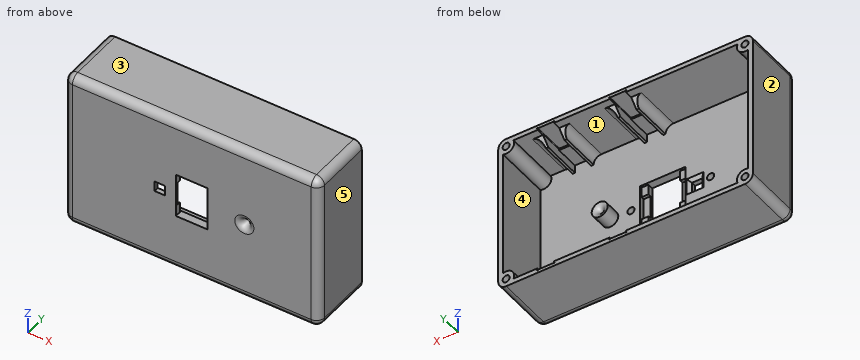
from build123d import *

# Parameters (mm, degrees)
SKETCH1_W                    = 160
SKETCH1_H                    = 100
MAINBODY_DEPTH               = 40
FILLET1_R                    = 5
SHELL1_START                 = 5
SHELL1_DEPTH                 = 35
ROTARYASSEMBLYCUTOUTSKETCH_W = 10.2
ROTARYASSEMBLYCUTOUTSKETCH_H = 20
ROTARYASSEMBLYCUTOUT_DEPTH   = 1
SKETCH5_R                    = 5
SCREWHOLEMATERIAL_DEPTH      = 35
SKETCH6_R                    = 2.25
INSERTHOLE_DEPTH             = 10
SKETCH8_W                    = 20
SKETCH8_H                    = 28
SCREENCUTOUT_DEPTH           = 101.623058987
SKETCH7_W                    = 28.6
SKETCH7_H                    = 28
SCREENCUTOUT1_DEPTH          = 1.4
SKETCH9_W                    = 28.6
SKETCH9_H                    = 15
SCREENCUTOUT2_DEPTH          = 2
SKETCH10_W                   = 6.5
SKETCH10_H                   = 6.5
BUTTONHOLE_DEPTH             = 101.623058987
SKETCH11_R                   = 2.25
HEATINSERTHOLE_DEPTH         = 4.2
SKETCH12_R                   = 5
STRINGSUPPORT_DEPTH          = 10
SKETCH13_R                   = 1
STRINGHOLE_DEPTH             = 98.59610648
FILLET2_R                    = 4
FILLET3_SIZE                 = 8
FILLET3_SIZE_2               = 5
SKETCH14_W                   = 1.5
SKETCH14_H                   = 30
BOSS_EXTRUDE1_DEPTH          = 5
SKETCH15_R                   = 0.5
CUT_EXTRUDE1_DEPTH           = 20
CHAMFER1_SIZE                = 5
FILLET5_R                    = 5
SKETCH17_W                   = 1.5
SKETCH17_H                   = 30
BOSS_EXTRUDE2_DEPTH          = 5
CHAMFER2_SIZE                = 5
FILLET6_R                    = 5
SKETCH16_R                   = 0.5
CUT_EXTRUDE2_DEPTH           = 20
SKETCH18_R                   = 0.375
CUT_EXTRUDE3_DEPTH           = 20
CHAMFER3_SIZE                = 2


# Read off the part's stored shape, not the designer's step: Shell1
# Some blends are built 0.0001 mm under size
with BuildPart() as part:
    # Sketch1 → MainBody (new body)
    with BuildSketch(Plane(origin=(0, 0, 0), x_dir=(1, 0, 0), z_dir=(0, 1, 0))):
        Rectangle(SKETCH1_W, SKETCH1_H)
    extrude(amount=MAINBODY_DEPTH)

    # Fillet1
    fillet1_edges = [part.edges().sort_by_distance(p)[0] for p in [
        (0, 0, -50),
        (80, 0, 0),
        (0, 0, 50),
        (-80, 0, 0),
        (-80, 20, -50),
        (80, 20, -50),
        (80, 20, 50),
        (-80, 20, 50),
    ]]
    fillet(fillet1_edges, radius=FILLET1_R)

    # Shell1 outline → Shell1 (cut)
    with BuildSketch(Plane(origin=(0, 0, 0), x_dir=(1, 0, 0), z_dir=(0, 1, 0)).offset(SHELL1_START)):
        with BuildLine():
            Line((-77, 45), (-77, -45))
            ThreePointArc((-77, -45), (-76.414213562, -46.414213562), (-75, -47))
            Line((-75, -47), (75, -47))
            ThreePointArc((75, -47), (76.414213562, -46.414213562), (77, -45))
            Line((77, -45), (77, 45))
            ThreePointArc((77, 45), (76.414213562, 46.414213562), (75, 47))
            Line((75, 47), (-75, 47))
            ThreePointArc((-75, 47), (-76.414213562, 46.414213562), (-77, 45))
        make_face()
    extrude(amount=SHELL1_DEPTH, mode=Mode.SUBTRACT)

    # RotaryAssemblyCutoutSketch → RotaryAssemblyCutout (cut)
    with BuildSketch(Plane(origin=(0, 0, 47), x_dir=(-1, 0, 0), z_dir=(0, 0, -1))):
        with Locations((-50.1, 30)):
            Rectangle(ROTARYASSEMBLYCUTOUTSKETCH_W, ROTARYASSEMBLYCUTOUTSKETCH_H)
        with Locations((-4.9, 30)):
            Rectangle(ROTARYASSEMBLYCUTOUTSKETCH_W, ROTARYASSEMBLYCUTOUTSKETCH_H)
    rotaryassemblycutout = extrude(amount=-ROTARYASSEMBLYCUTOUT_DEPTH, mode=Mode.SUBTRACT)

    # CutoutMirror: RotaryAssemblyCutout across plane
    add(rotaryassemblycutout.mirror(Plane(origin=(0, 0, 0), x_dir=(1, 0, 0), z_dir=(0, 0, -1))), mode=Mode.SUBTRACT)

    # Sketch5 → ScrewHoleMaterial (add)
    with BuildSketch(Plane(origin=(0, 40, 0), x_dir=(1, 0, 0), z_dir=(0, 1, 0))):
        with Locations((-75, 45)):
            Circle(SKETCH5_R)
        with Locations((-75, -45)):
            Circle(SKETCH5_R)
        with Locations((75, -45)):
            Circle(SKETCH5_R)
        with Locations((75, 45)):
            Circle(SKETCH5_R)
    extrude(amount=-SCREWHOLEMATERIAL_DEPTH)

    # Sketch6 → InsertHole (cut)
    with BuildSketch(Plane(origin=(0, 40, 0), x_dir=(1, 0, 0), z_dir=(0, 1, 0))):
        with Locations(Location((-75, 45, 0), (0, 0, 270))):
            Circle(SKETCH6_R)
        with Locations(Location((-75, -45, 0), (0, 0, 270))):
            Circle(SKETCH6_R)
        with Locations(Location((75, -45, 0), (0, 0, 270))):
            Circle(SKETCH6_R)
        with Locations(Location((75, 45, 0), (0, 0, 270))):
            Circle(SKETCH6_R)
    extrude(amount=-INSERTHOLE_DEPTH, mode=Mode.SUBTRACT)

    # Sketch8 → ScreenCutout (cut, through all)
    with BuildSketch(Plane(origin=(0, 5, 0), x_dir=(1, 0, 0), z_dir=(0, 1, 0))):
        Rectangle(SKETCH8_W, SKETCH8_H)
    extrude(amount=-SCREENCUTOUT_DEPTH, mode=Mode.SUBTRACT)

    # Sketch7 → ScreenCutout1 (cut)
    with BuildSketch(Plane(origin=(0, 5, 0), x_dir=(1, 0, 0), z_dir=(0, 1, 0))):
        Rectangle(SKETCH7_W, SKETCH7_H)
    extrude(amount=-SCREENCUTOUT1_DEPTH, mode=Mode.SUBTRACT)

    # Sketch9 → ScreenCutout2 (cut)
    with BuildSketch(Plane(origin=(0, 3.6, 0), x_dir=(1, 0, 0), z_dir=(0, 1, 0))):
        Rectangle(SKETCH9_W, SKETCH9_H)
    extrude(amount=-SCREENCUTOUT2_DEPTH, mode=Mode.SUBTRACT)

    # Sketch10 → ButtonHole (cut, through all)
    with BuildSketch(Plane(origin=(0, 5, 0), x_dir=(1, 0, 0), z_dir=(0, 1, 0))):
        with Locations((-20.2, 0)):
            Rectangle(SKETCH10_W, SKETCH10_H)
    extrude(amount=-BUTTONHOLE_DEPTH, mode=Mode.SUBTRACT)

    # Sketch11 → HeatInsertHole (cut)
    with BuildSketch(Plane(origin=(0, 5, 0), x_dir=(1, 0, 0), z_dir=(0, 1, 0))):
        with Locations(Location((-30, 0, 0), (0, 0, 270))):
            Circle(SKETCH11_R)
        with Locations(Location((20, 0, 0), (0, 0, 270))):
            Circle(SKETCH11_R)
    extrude(amount=-HEATINSERTHOLE_DEPTH, mode=Mode.SUBTRACT)

    # Sketch12 → StringSupport (add)
    with BuildSketch(Plane(origin=(0, 5, 0), x_dir=(1, 0, 0), z_dir=(0, 1, 0))):
        with Locations(Location((33, 0, 0), (0, 0, 270))):
            Circle(SKETCH12_R)
    extrude(amount=STRINGSUPPORT_DEPTH)

    # Sketch13 → StringHole (cut, through all)
    with BuildSketch(Plane(origin=(0, 15, 0), x_dir=(1, 0, 0), z_dir=(0, 1, 0))):
        with Locations(Location((33, 0, 0), (0, 0, 270))):
            Circle(SKETCH13_R)
    extrude(amount=-STRINGHOLE_DEPTH, mode=Mode.SUBTRACT)

    # Fillet2
    fillet2_edges = [part.edges().sort_by_distance(p)[0] for p in [
        (33, 15, -1),
    ]]
    fillet(fillet2_edges, radius=FILLET2_R - 0.0001)  # a hair under: the kernel refuses the full size

    # Fillet3
    # an asymmetric fillet: 8, 5 mm, written as the material it takes off along each edge
    with BuildSketch(Plane(origin=(33, 0, 0), x_dir=(0, 0, 1), z_dir=(-1, 0, 0))) as fillet3_piece_1:
        with BuildLine():
            Bezier((1, FILLET3_SIZE), (1, 0), (1 + FILLET3_SIZE_2, 0), weights=[1, 0.707106781, 1])
            Line((1 + FILLET3_SIZE_2, 0), (1, 0))
            Line((1, 0), (1, FILLET3_SIZE))
        make_face()
    revolve(axis=Axis((33, 0, 0), (0, 1, 0)), mode=Mode.SUBTRACT)

    # Sketch14 → Boss-Extrude1 (add)
    with BuildSketch(Plane.XY.offset(-47)):
        with Locations((-0.95, 20)):
            Rectangle(SKETCH14_W, SKETCH14_H)
        with Locations((10.75, 20)):
            Rectangle(SKETCH14_W, SKETCH14_H)
    extrude(amount=BOSS_EXTRUDE1_DEPTH)

    # Sketch15 → Cut-Extrude1 (cut)
    with BuildSketch(Plane(origin=(0, 40, 0), x_dir=(1, 0, 0), z_dir=(0, 1, 0))):
        with Locations((-0.2, 48)):
            Circle(SKETCH15_R)
        with Locations((10, 48)):
            Circle(SKETCH15_R)
    extrude(amount=-CUT_EXTRUDE1_DEPTH, mode=Mode.SUBTRACT)

    # Chamfer1
    chamfer1_edges = [part.edges().sort_by_distance(p)[0] for p in [
        (10.75, 35, -42),
        (-0.95, 35, -42),
    ]]
    chamfer(chamfer1_edges, length=CHAMFER1_SIZE - 0.0001)  # a hair under: the kernel refuses the full size

    # Fillet5
    # the kernel refuses this fillet: 5 mm, written as the material it adds along each edge
    with BuildSketch(Plane(origin=(11.5, 5, -47), x_dir=(0, 0, 1), z_dir=(0, 1, 0))) as fillet5_piece_1_section:
        with BuildLine():
            CenterArc((FILLET5_R, FILLET5_R), FILLET5_R, 180, 90)
            Line((0, FILLET5_R), (0, 0))
            Line((0, 0), (FILLET5_R, 0))
        make_face()
    fillet5_piece_1 = extrude(amount=42.5, mode=Mode.PRIVATE)
    fillet5_piece_1 = split(fillet5_piece_1, bisect_by=Plane(origin=(12.655573562, 26.680118084, -38.680018084), z_dir=(0, -0.7071067811865479, -0.7071067811865474)), keep=Keep.TOP, mode=Mode.PRIVATE)
    add(fillet5_piece_1)
    with BuildSketch(Plane(origin=(-1.7, 47.5, -47), x_dir=(-1, 0, 0), z_dir=(0, -1, 0))) as fillet5_piece_2_section:
        with BuildLine():
            CenterArc((FILLET5_R, -FILLET5_R), FILLET5_R, 90, 90)
            Line((0, -FILLET5_R), (0, 0))
            Line((0, 0), (FILLET5_R, 0))
        make_face()
    fillet5_piece_2 = extrude(amount=42.5, mode=Mode.PRIVATE)
    fillet5_piece_2 = split(fillet5_piece_2, bisect_by=Plane(origin=(-4.149999992, 35.05005, -47.04995), z_dir=(0, -0.7071067811865479, -0.7071067811865474)), keep=Keep.TOP, mode=Mode.PRIVATE)
    add(fillet5_piece_2)

    # Sketch17 → Boss-Extrude2 (add)
    with BuildSketch(Plane.XY.offset(-47)):
        with Locations((44.25, 20)):
            Rectangle(SKETCH17_W, SKETCH17_H)
        with Locations((55.95, 20)):
            Rectangle(SKETCH17_W, SKETCH17_H)
    extrude(amount=BOSS_EXTRUDE2_DEPTH)

    # Chamfer2
    chamfer2_edges = [part.edges().sort_by_distance(p)[0] for p in [
        (55.95, 35, -42),
        (44.25, 35, -42),
    ]]
    chamfer(chamfer2_edges, length=CHAMFER2_SIZE - 0.0001)  # a hair under: the kernel refuses the full size

    # Fillet6
    # the kernel refuses this fillet: 5 mm, written as the material it adds along each edge
    with BuildSketch(Plane(origin=(56.7, 47.5, -47), x_dir=(0, 0, 1), z_dir=(0, -1, 0))) as fillet6_piece_1_section:
        with BuildLine():
            CenterArc((FILLET6_R, -FILLET6_R), FILLET6_R, 90, 90)
            Line((0, -FILLET6_R), (0, 0))
            Line((0, 0), (FILLET6_R, 0))
        make_face()
    fillet6_piece_1 = extrude(amount=42.5, mode=Mode.PRIVATE)
    fillet6_piece_1 = split(fillet6_piece_1, bisect_by=Plane(origin=(59.149999992, 35.05005, -47.04995), z_dir=(0, -0.7071067811865479, -0.7071067811865474)), keep=Keep.TOP, mode=Mode.PRIVATE)
    add(fillet6_piece_1)
    with BuildSketch(Plane(origin=(43.5, 47.5, -47), x_dir=(0, 0, 1), z_dir=(0, -1, 0))) as fillet6_piece_2_section:
        with BuildLine():
            CenterArc((FILLET6_R, FILLET6_R), FILLET6_R, 180, 90)
            Line((0, FILLET6_R), (0, 0))
            Line((0, 0), (FILLET6_R, 0))
        make_face()
    fillet6_piece_2 = extrude(amount=42.5, mode=Mode.PRIVATE)
    fillet6_piece_2 = split(fillet6_piece_2, bisect_by=Plane(origin=(41.050000008, 35.05005, -47.04995), z_dir=(0, -0.7071067811865479, -0.7071067811865474)), keep=Keep.TOP, mode=Mode.PRIVATE)
    add(fillet6_piece_2)

    # Sketch16 → Cut-Extrude2 (cut)
    with BuildSketch(Plane(origin=(0, 40, 0), x_dir=(1, 0, 0), z_dir=(0, 1, 0))):
        with Locations((45, 48)):
            Circle(SKETCH16_R)
        with Locations((55.2, 48)):
            Circle(SKETCH16_R)
    extrude(amount=-CUT_EXTRUDE2_DEPTH, mode=Mode.SUBTRACT)

    # Mirror5: part across plane


with BuildPart() as part_1:
    add(part.part)
    add(part.part.mirror(Plane.XY))

    # Sketch18 → Cut-Extrude3 (cut)
    with BuildSketch(Plane(origin=(0, 40, 0), x_dir=(1, 0, 0), z_dir=(0, 1, 0))):
        with Locations((-0.2, 48)):
            Circle(SKETCH18_R)
        with Locations((10, 48)):
            Circle(SKETCH18_R)
        with Locations((45, 48)):
            Circle(SKETCH18_R)
        with Locations((55.2, 48)):
            Circle(SKETCH18_R)
        with Locations((-0.2, -48)):
            Circle(SKETCH18_R)
        with Locations((10, -48)):
            Circle(SKETCH18_R)
        with Locations((45, -48)):
            Circle(SKETCH18_R)
        with Locations((55.2, -48)):
            Circle(SKETCH18_R)
    extrude(amount=-CUT_EXTRUDE3_DEPTH, mode=Mode.SUBTRACT)

    # Chamfer3
    chamfer3_edges = [part_1.edges().sort_by_distance(p)[0] for p in [
        (-23.45, 5, 0),
        (-20.2, 5, 3.25),
        (-16.95, 5, 0),
        (-20.2, 5, -3.25),
    ]]
    chamfer(chamfer3_edges, length=CHAMFER3_SIZE)


solid = part_1.part
For this review, take the finished solid that the model builds, in its own axes (mm). Face numbers are marked on the shaded views. A direction names the side the tool comes from. Round coordinates to 2 decimals unless told otherwise and drop trailing zeros. Loops run counter-clockwise (first coordinate to the right, second up) from the corner with the lowest first, then second, coordinate; pieces in that order, holes last. Notation, with made-up numbers: (78.5, 1.25) - (92.5, 1.25) arc R16 ccw to (92.5, 22.25) - close; hole circle Ø9 at (6, 53). An arc over 180 degrees is marked (long way). One line per question, with ' | ' between items.
Q1. Take a section at B-B (x = 20). Give the boundary of the cut face in (y, z).
Taken from the geometry:
outline: (0, -45) arc R5 ccw to (5, -50) - (40, -50) - (40, -47) - (5, -47) - (5, -2.25) - (0.8, -2.25) - (0.8, 2.25) - (5, 2.25) - (5, 47) - (40, 47) - (40, 50) - (5, 50) arc R5 ccw to (0, 45) - close
Q2. For line 1 along X through (y, z) = (37.25, 45); line 2 along Z through (x, y) = (63.5, 21); line 3 along X through (y, z) = (37, -18.5), list the stretches that pass through material, from the lowest coordinate up. Write a range as [from, to].
Taken from the geometry:
line 1: x = [-80, -77.25], [-72.75, -70], [70, 72.75], [77.25, 80] | line 2: z = [-50, -47], [47, 50] | line 3: x = [-80, -77], [77, 80]
Q3. Tool access review of the marked faces 4 and 5: name each direction out of +Z, -Z, +X, -X, +Y, -Y from which nothing blocks a thin tool from reaching the whole face with its end or side.
Taken from the geometry:
face 4: +Y | face 5: +Z, -Z, +X, +Y, -Y
Q4. The part is to be moulded in two halves that separate along X. For the marked faces 1, 2 and 3, say which applies: released by +X, released by -X, zero draft, split by the parting line, or undercut.
Taken from the geometry:
face 1: undercut | face 2: released by -X | face 3: zero draft
Q5. Take a section at A-A (x = 3.5). Give the boundary of the cut face in (y, z).
Taken from the geometry:
outline: (0, -45) arc R5 ccw to (5, -50) - (40, -50) - (40, -48) - (20, -48) - (20, -47) - (5, -47) - (5, -14) - (0, -14) - close; (0, 14) - (5, 14) - (5, 47) - (20, 47) - (20, 48) - (40, 48) - (40, 50) - (5, 50) arc R5 ccw to (0, 45) - close
Q6. For pin 1 (10 mm diameter, centred on x = 29.5, z = 39.5, fed in from +Y); pin 2 (0.6 mm diameter, centred on x = 11.5, y = 2, fed in from -Z); pin 3 (1.3 mm diameter, centred on x = -11, z = 3, fed in from +Y), all flat-tipped, find the tip position at first contact; note any pin that passes through.
Taken from the geometry:
pin 1: stops at y = 5 | pin 2: stops at z = -49.21 | pin 3: stops at y = 1.6
Q7. Take a section at C-C (x = -67.5). Give the boundary of the cut face in (y, z), and give its area (3 significant figures).
Taken from the geometry:
outline: (0, -45) arc R5 ccw to (5, -50) - (40, -50) - (40, -47) - (5, -47) - (5, 47) - (40, 47) - (40, 50) - (5, 50) arc R5 ccw to (0, 45) - close | area: 699 mm²
